Verification items for this drawing (mm, ordinates from the low corner). A direction names the side the tool comes from. Round coordinates to 2 decimals unless told otherwise and drop trailing zeros. Write each loop counter-clockwise with the first axis right and the second up, starting at its lowest first coordinate (ties: lowest second). Pieces come first, ordered by that corner, then holes. Notation, with made-up numbers: (16.5, 25.25) -> (51.5, 25.25) arc R13 ccw to (51.5, 49.25) -> close; hole circle Ø5 at (31, -27). An arc over 180 degrees is marked (long way). Use one line per item in the form item = value. Start each with the question number.
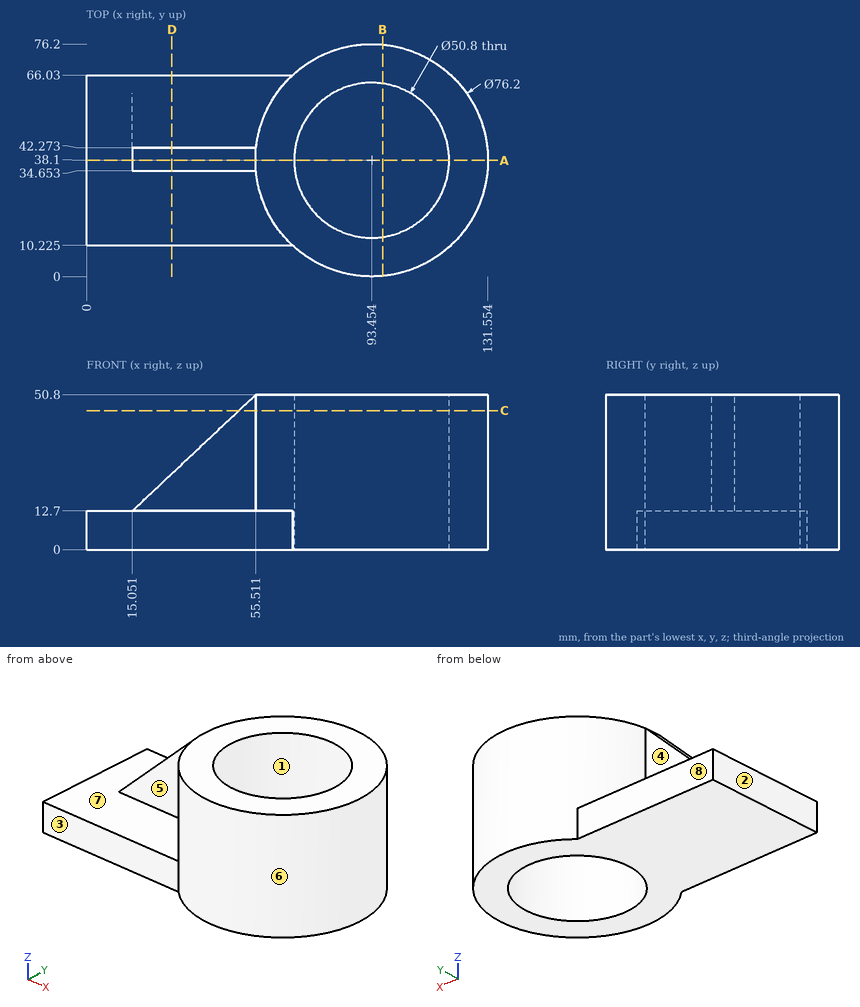
1. Sectioned sample at D-D (x = 28). Enter the section's corners in (y, z) (1 decimal).
2. Depth check by flat-ended pin: pin 1 (6 mm diameter, centred on x = 102, z = 24, fed in from +Y); pin 2 (4 mm diameter, centred on x = 41, z = 4, fed in from -Y) (1 decimal); pin 3 (12 mm diameter, centred on x = 48, z = 30, fed in from +Y). Enter the tip coordinate at first touch or a pass-through.
3. Scan lines: probe 1 along X at (y, z) = (38, 12) (1 decimal); probe 2 along X at (y, z) = (37.5, 8.5); probe 3 along Z at (x, y) = (62, 12.5). Record each from-to range of solid material in increasing order.
4. Sectioned sample at B-B (x = 97). Enter the section's corners in (y, z) (1 decimal), and give its area (3 significant figures).
5. Sectioned sample at A-A (y = 38.1). Enter the section's corners in (x, z) (1 decimal), and give its area (3 significant figures).
6. Tool access check on the marked faces 4, 5, 6, 7 and 8. Record the directions out of +Z, -Z, +X, -X, +Y, -Y that give a thin tool (end or side, any length) a straight path to the whole face; none if there is none.
7. Sectioned sample at C-C (z = 45.5). Enter the section's corners in (x, y) (1 decimal), and give its area (3 significant figures).
8. Mould release check, pull along Y, two halves, no side actions. Record for the marked faces 1, 2 and 3: +Y half, -Y half, draft (parallel to the pull), parting line (faces both ways), or undercut.
Returned:
q1.outline = (10.2, 0) -> (66, 0) -> (66, 12.7) -> (42.3, 12.7) -> (42.3, 24.9) -> (34.7, 24.9) -> (34.7, 12.7) -> (10.2, 12.7) -> close
q2.pin_1 = 75.79
q2.pin_2 = 10.2
q2.pin_3 = 42.27
q3.probe_1 = 0 to 68.1, 118.9 to 131.6
q3.probe_2 = 0 to 68.06, 118.85 to 131.55
q3.probe_3 = 0 to 12.7
q4.outline = (0.2, 0) -> (12.9, 0) -> (12.9, 50.8) -> (0.2, 50.8) -> close; (63.3, 0) -> (76, 0) -> (76, 50.8) -> (63.3, 50.8) -> close
q4.area = 1,300 mm^2
q5.outline = (0, 0) -> (68.1, 0) -> (68.1, 50.8) -> (55.5, 50.8) -> (15.1, 12.7) -> (0, 12.7) -> close; (118.9, 0) -> (131.6, 0) -> (131.6, 50.8) -> (118.9, 50.8) -> close
q5.area = 2,760 mm^2
q6.face_4 = +Z, -X, +Y
q6.face_5 = +Z, -X, -Y
q6.face_6 = +Z
q6.face_7 = +Z, -X
q6.face_8 = +Z, -Z, -X, +Y
q7.outline = (49.9, 34.7) -> (55.5, 34.7) arc R38.1 ccw (long way) to (55.6, 42.3) -> (49.9, 42.3) -> close; hole circle Ø50.8 at (93.5, 38.1)
q7.area = 2,580 mm^2
q8.face_1 = undercut
q8.face_2 = draft
q8.face_3 = -Y half
